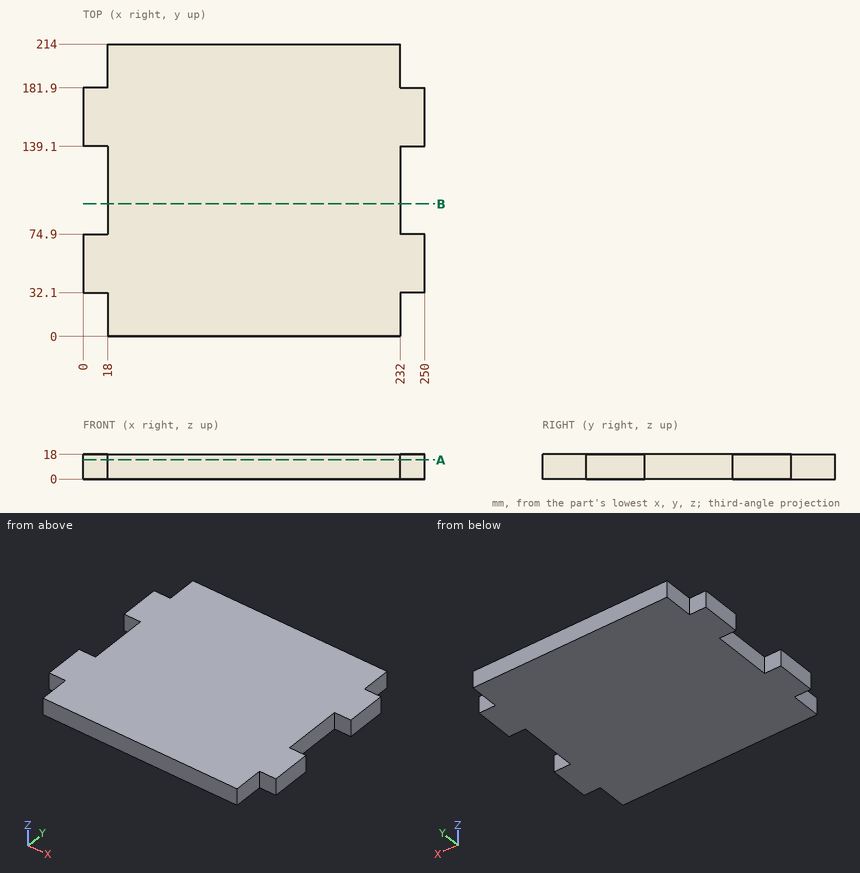
Answer from the drawing. Dimensions are ordinates in mm from the lowest x, y and z of the part. Round coordinates to 2 decimals unless told otherwise and drop trailing zeros. Write each loop counter-clockwise with the first axis right and the second up, starting at its lowest first coordinate (ties: lowest second). Pieces come first, ordered by that corner, then holes.
1. The part is cut by section A-A, the plane z = 14. Determine the outline of the cut face in (x, y).
2. The part is cut by section B-B, the plane y = 97. Determine the outline of the cut face in (x, z), then the cut area to 3 significant figures.
3. Straight lines are drawn through the part: L1, parallel to Y at x = 15.5, z = 12.75; L2, parallel to X at y = 13, z = 9.25. For each, find the intervals that lie inside material, in ascending order.
4. Given pin 1 Ø9 at (x, z) = (237.5, 6.5) entering from -Y; pin 2 Ø9 at (y, z) = (17.5, 8) entering from -X; pin 3 Ø2 at (y, z) = (170, 8) entering from -X; pin 4 Ø9 at (y, z) = (17, 10.5) entering from +X, each flat-ended and moving along its own axis, determine where each tip first touches the part or whether it passes through.
Values:
1. outline: (0, 32.1) - (18, 32.1) - (18, 0) - (232, 0) - (232, 32.1) - (250, 32.1) - (250, 74.9) - (232, 74.9) - (232, 139.1) - (250, 139.1) - (250, 181.9) - (232, 181.9) - (232, 214) - (18, 214) - (18, 181.9) - (0, 181.9) - (0, 139.1) - (18, 139.1) - (18, 74.9) - (0, 74.9) - close
2. outline: (18, 0) - (232, 0) - (232, 18) - (18, 18) - close
2. area: 3,850 mm2
3. L1: y = 32.1 to 74.9, 139.1 to 181.9
3. L2: x = 18 to 232
4. pin 1: stops at y = 32.1
4. pin 2: stops at x = 18
4. pin 3: stops at x = 0
4. pin 4: stops at x = 232
